Autodesk Inventor part; units mm, degrees
ref_plane "YZ Plane" through (0, 0, 0) normal (1, 0, 0) x (0, 1, 0)
ref_plane "XZ Plane" through (0, 0, 0) normal (0, 1, 0) x (-1, 0, 0)
ref_plane "XY Plane" through (0, 0, 0) normal (0, 0, 1) x (1, 0, 0)
sketch "Sketch1" plane through (0, 0, 0) normal (1, 0, 0) x (0, 1, 0)
  line L0 (0, 1.5838) -> (0, -3.1787)
  line L1 (-2.7424, -3.1787) -> (-5.4957, 1.5775)
  line L2 (-5.4957, 1.5775) -> (-2.7532, 6.34)
  line L3 (-2.7532, 6.34) -> (2.7424, 6.3463)
  line L4 (2.7424, 6.3463) -> (5.4957, 1.59)
  line L5 (5.4957, 1.59) -> (2.7532, -3.1725)
  line L6 (2.7532, -3.1725) -> (-2.7424, -3.1787)
  point P0 (0, 0)
  dimension "d0" = 4.7625
extrude "Extrusion1" add sketch "Sketch1" along normal blind 34.29
sketch "Sketch2" plane through (34.29, 0, 0) normal (1, 0, 0) x (0, 0, -1)
  line L0 (3.1725, 2.7532) -> (-1.59, 5.4957)
  line L1 (0.7913, 4.1244) -> (-1.5775, -0.0072)
  circle A0 centre (-1.5775, -0.0072) radius 4.7625
  point P0 (0, 0)
  dimension "d3" = 4.7625
extrude "Extrusion2" add sketch "Sketch2" along normal blind 6.35
sketch "Sketch3" plane through (0, 0, 0) normal (-1, 0, 0) x (0, 0, 1)
  line L0 (-1.0999, -3.9458) -> (-3.1787, -2.7424) construction
  arc A0 (4.1618, -4.0075) -> (-0.799, 4.12) centre (1.5775, -0.0072) ccw construction
  line L1 (-1.0999, -3.9458) -> (1.5775, -0.0072) construction
  circle A1 centre (1.5775, -0.0072) radius 4.7625
  point P0 (0, 0)
  dimension "d6" = 4.7625
extrude "Extrusion3" add sketch "Sketch3" along normal blind 6.35
properties part number "Hex Shaft"
The model under review builds one solid part; all positions refer to its coordinate system, in mm. A direction names the side the tool comes from. Round coordinates to 2 decimals unless told otherwise and drop trailing zeros. Loops run counter-clockwise (first coordinate to the right, second up) from the corner with the lowest first, then second, coordinate; pieces in that order, holes last. Notation, with made-up numbers: (-11.5, 41.25) -> (17.5, 41.25) arc R17 ccw to (17.5, 72.25) -> close; hole circle Ø9 at (40, -22). An arc over 180 degrees is marked (long way). Write item = value, one per line. Start each with the question number.
Item 1: Insertion check: pin 1 (1.5 mm diameter, centred on x = 21.5, y = -1.5, fed in from +Z); pin 2 (1 mm diameter, centred on x = 21.5, z = 5, fed in from +Y). Each pin has a flat end and moves straight along its axis. Give the tip position at first contact, or say it passes through.
Item 2: Take a section at A-A on x = 21. Give the boundary of the cut face in (y, z), plus the area to 3 significant figures.
Item 3: Take a section at C-C on z = 1. Give the boundary of the cut face in (x, y).
Item 4: To check wall thickness, follow L1, parallel to Z at x = 18.5, y = -0.75; L2, parallel to Y at x = 30, z = 3.25; L3, parallel to Z at x = 9.5, y = 4.75. State the ranges of each line that lie inside material, in increasing order.
Item 5: Take a section at B-B on y = -1.75. Give the boundary of the cut face in (x, z).
Item 6: For faces 1 (the flat face through (0, 2, -3)), 2 (the cylindrical face through (-3.13, -3.23, -1.93)), 3 (the flat face through (34.29, 2, -3)), 4 (the flat face through (34.29, -2.5, -2.7)), list the 3-axis set-ups (+Z, -Z, +X, -X, +Y, -Y) from which the entire face can be reached by the end or side of a thin tool; tool diameter is ignored.
Result:
q1.pin_1 = 6.34
q1.pin_2 = 3.81
q2.outline = (-5.5, 1.58) -> (-2.74, -3.18) -> (2.75, -3.17) -> (5.5, 1.59) -> (2.74, 6.35) -> (-2.75, 6.34) -> close
q2.area = 78.5 mm²
q3.outline = (-6.35, -4.73) -> (0, -4.73) -> (0, -5.16) -> (34.29, -5.16) -> (34.29, -4.73) -> (40.64, -4.73) -> (40.64, 4.72) -> (34.29, 4.72) -> (34.29, 5.16) -> (0, 5.16) -> (0, 4.72) -> (-6.35, 4.72) -> close
q4.L1 = -3.18 to 6.34
q4.L2 = -4.53 to 4.53
q4.L3 = 0.3 to 2.88
q5.outline = (-6.35, -2.85) -> (0, -2.85) -> (0, -3.18) -> (34.29, -3.18) -> (34.29, -2.85) -> (40.64, -2.85) -> (40.64, 6.01) -> (34.29, 6.01) -> (34.29, 6.34) -> (0, 6.34) -> (0, 6.01) -> (-6.35, 6.01) -> close
q6.face_1 = -Z, -X, +Y
q6.face_2 = -X
q6.face_3 = -Z, +X, +Y
q6.face_4 = -Z, +X, -Y
